Here's how the part is built. I have some questions about the finished solid (model axes, mm). A direction names the side the tool comes from. Coordinates: 2 decimals unless noted, no trailing zeros. Loops run counter-clockwise (first coordinate to the right, second up) from the corner with the lowest first, then second, coordinate; pieces in that order, holes last. Notation, with made-up numbers: M 67.5,-9.5 L 93.5,-9.5 A12 ccw 93.5,11.5 Z; hole C 33.25,73 d11. An arc over 180 degrees is marked long. Use one line per item in the form item = value. Start each with the question number.
(1) Imagine slicing it at D-D, the plane z = -58. Please give me the cut outline in (x, y), and give its area (3 significant figures).
(2) Please list where these lines run through material, in increasing order: L1, parallel to Z at x = 10, y = 17.75; L2, parallel to Z at x = -28.5, y = 17; L3, parallel to X at y = 16.5, z = 49.5.
(3) Imagine slicing it at B-B, the plane x = 32. Please give me the cut outline in (y, z), and give its area (3 significant figures).
(4) Will these pins go through, and if not, where does the flat tip stop? P1, Ø2.5, axis at x = -33.5, y = 10, coming from the +Z side; P2, Ø1, axis at x = -28.5, z = 57, coming from the +Y side; P3, Ø1.6, axis at x = 23.5, y = 1, coming from the +Z side.
(5) On a 3-axis mill with a long thin cutter (end or side, diameter ignored), from which of +Z, -Z, +X, -X, +Y, -Y can I reach the whole of each face in a straight line? I mean faces 1 (the flat face through (-28, 2, -3)), 2 (the flat face through (-28.314, 10, 58)), 3 (the flat face through (10, 18, 46.703)), 4 (the flat face through (-33, 19, 58)), 5 (the flat face through (28, 2, 1)). Say none if no direction works.
(6) Thinking about a two-plate mould opening in Z: for faces 6 (the flat face through (-38, 18, 46.703)), 7 (the flat face through (20, 10, 78.719)), 8 (the flat face through (-1, 20, -54)), which applies, +Z half, -Z half, draft (parallel to the pull), parting line (faces both ways), or undercut?
(7) Imagine slicing it at C-C, the plane y = 17. Please give me the cut outline in (x, z), and give its area (3 significant figures).
(8) Imagine slicing it at A-A, the plane z = 66. Please give me the cut outline in (x, y), and give its area (3 significant figures).
```python
from build123d import *

# Parameters (mm, degrees)
SKETCH1_W           = 121.603901538
SKETCH1_H           = 157.438867692
BOSS_EXTRUDE1_DEPTH = 20
SKETCH2_W           = 17.97576728
SKETCH2_H           = 23.568228212
SKETCH2_W_2         = 17.951314889
SKETCH2_H_2         = 23.536168411
CUT_EXTRUDE1_DEPTH  = 1
SKETCH3_W           = 95.285802818
SKETCH3_H           = 93.40563605
CUT_EXTRUDE2_DEPTH  = 5
SKETCH5_W           = 18.1
SKETCH5_H           = 157.438867692
CUT_EXTRUDE3_DEPTH  = 2
SKETCH6_W           = 2
SKETCH6_H           = 18
CUT_EXTRUDE4_DEPTH  = 33
SKETCH8_W           = 18.1
SKETCH8_H           = 18
CUT_EXTRUDE5_DEPTH  = 8.45273398


with BuildPart() as part:
    # Sketch1 → Boss-Extrude1 (new body)
    with BuildSketch(Plane(origin=(0, 0, 0), x_dir=(1, 0, 0), z_dir=(0, 1, 0))):
        Rectangle(SKETCH1_W, SKETCH1_H)
    extrude(amount=BOSS_EXTRUDE1_DEPTH)

    # Sketch2 → Cut-Extrude1 (cut)
    with BuildSketch(Plane(origin=(0, 20, 0), x_dir=(1, 0, 0), z_dir=(0, 1, 0))):
        with Locations((-27.924267606, -58.48258576)):
            Rectangle(SKETCH2_W, SKETCH2_H)
        with Locations((28.722103823, -58.283126705)):
            Rectangle(SKETCH2_W_2, SKETCH2_H_2)
    extrude(amount=-CUT_EXTRUDE1_DEPTH, mode=Mode.SUBTRACT)

    # Sketch3 → Cut-Extrude2 (cut)
    with BuildSketch(Plane(origin=(0, 20, 0), x_dir=(1, 0, 0), z_dir=(0, 1, 0))):
        Rectangle(SKETCH3_W, SKETCH3_H)
    extrude(amount=-CUT_EXTRUDE2_DEPTH, mode=Mode.SUBTRACT)

    # Sketch5 → Cut-Extrude3 (cut)
    with BuildSketch(Plane.XZ):
        with Locations((-28.163629981, 0)):
            Rectangle(SKETCH5_W, SKETCH5_H)
        with Locations((28.080400305, 0.136730642)):
            Rectangle(SKETCH5_W, SKETCH5_H)
    extrude(amount=-CUT_EXTRUDE3_DEPTH, mode=Mode.SUBTRACT)

    # Sketch6 → Cut-Extrude4 (cut)
    with BuildSketch(Plane(origin=(-36.912151246, 20, 46.702818025), x_dir=(1, 0, 0), z_dir=(0, 0, 1))):
        with Locations((9.598521265, -9)):
            Rectangle(SKETCH6_W, SKETCH6_H)
    extrude(amount=CUT_EXTRUDE4_DEPTH, mode=Mode.SUBTRACT)

    # Sketch8 → Cut-Extrude5 (cut)
    with BuildSketch(Plane.XY.offset(78.719433846)):
        with Locations((-28.163629981, 11)):
            Rectangle(SKETCH8_W, SKETCH8_H)
    extrude(amount=-CUT_EXTRUDE5_DEPTH, mode=Mode.SUBTRACT)


solid = part.part
```
Answer:
q1.outline = M -60.8,0 L -37.21,0 L -37.21,2 L -19.11,2 L -19.11,0 L 19.03,0 L 19.03,2 L 37.13,2 L 37.13,0 L 60.8,0 L 60.8,20 L -60.8,20 Z
q1.area = 2,360 mm²
q2.L1 = -78.72 to -46.7, 46.7 to 78.72
q2.L2 = -78.72 to -46.7, 46.7 to 70.27
q2.L3 = -60.8 to -28.31, -26.31 to 60.8
q3.outline = M 0,-78.72 L 20,-78.72 L 20,-46.7 L 15,-46.7 L 15,46.7 L 19,46.7 L 19,70.05 L 20,70.05 L 20,78.72 L 2,78.72 L 2,-78.58 L 0,-78.58 Z
q3.area = 2,340 mm²
q4.P1 = 70.27
q4.P2 = 19
q4.P3 = -78.58
q5.face_1 = +Z, -Z, -Y
q5.face_2 = +Z, +Y, -Y
q5.face_3 = +Y
q5.face_4 = +Z, +Y
q5.face_5 = +Z, -Y
q6.face_6 = undercut
q6.face_7 = +Z half
q6.face_8 = draft
q7.outline = M -60.8,-78.72 L 60.8,-78.72 L 60.8,78.72 L -19.11,78.72 L -19.11,70.27 L -26.31,70.27 L -26.31,46.7 L 47.64,46.7 L 47.64,-46.7 L -47.64,-46.7 L -47.64,46.7 L -28.31,46.7 L -28.31,70.27 L -37.21,70.27 L -37.21,78.72 L -60.8,78.72 Z
q7.area = 10,000 mm²
q8.outline = M -60.8,0 L -37.21,0 L -37.21,2 L -28.31,2 L -28.31,19 L -36.91,19 L -36.91,20 L -60.8,20 Z; M -26.31,2 L -19.11,2 L -19.11,0 L 19.03,0 L 19.03,2 L 37.13,2 L 37.13,0 L 60.8,0 L 60.8,20 L 37.7,20 L 37.7,19 L 19.75,19 L 19.75,20 L -18.94,20 L -18.94,19 L -26.31,19 Z
q8.area = 2,290 mm²
